For this review, use the dimensioned drawing (mm, ordinates from the lowest corner) and the shaded views. Coordinates: 2 decimals unless noted, no trailing zeros. Write each loop counter-clockwise with the first axis right and the second up, starting at its lowest first coordinate (ties: lowest second). Pieces come first, ordered by that corner, then holes. Notation, with made-up numbers: M 37,-0.5 L 83,-0.5 A29 ccw 83,20.5 Z; hole C 41.25,-34 d8. An arc over 180 degrees is marked long. Return JSON: item names as keys, results as strings. Group by question number.
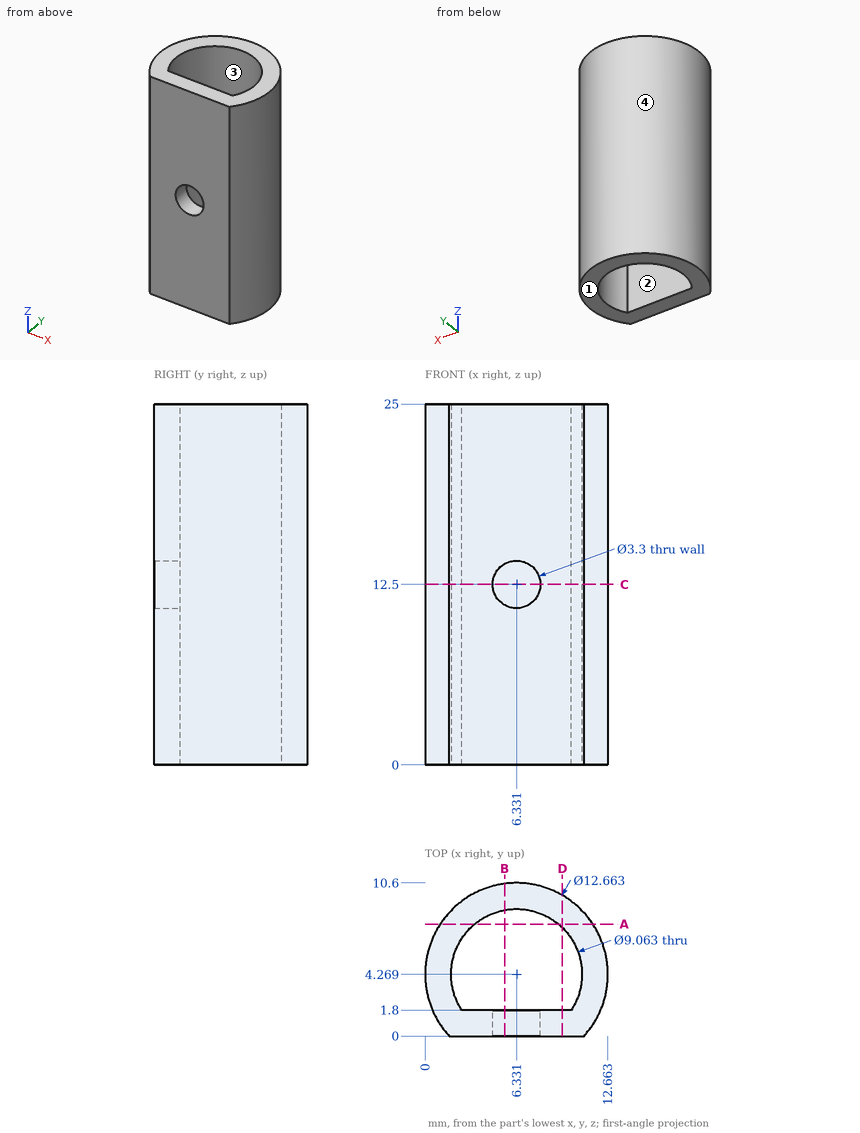
Item 1: The part is to be moulded in two halves that separate along X. For the marked faces 1, 2, 3 and 4, say which applies: pulls with the +X half, pulls with the -X half, needs draft (parallel to the pull), parting line crosses it, or undercut.
Item 2: For pin 1 (1 mm diameter, centred on y = 3, z = 8, fed in from -X), flat-tipped, find the tip position at first contact; note if it passes through.
Item 3: Add section A-A (y = 7.75). Write out the cut boundary in (x, z), plus the area to 3 significant figures.
Item 4: Add section C-C (z = 12.5). Write out the cut boundary in (x, y) (1 decimal).
Item 5: Add section D-D (x = 9.5). Write out the cut boundary in (y, z), plus the area to 3 significant figures.
Item 6: Add section B-B (x = 5.5). Write out the cut boundary in (y, z) (1 decimal).
Item 7: For line 1 (X direction, y = 3.25, z = 17.25) (1 decimal); line 2 (X direction, y = 7.5, z = 21.25) (1 decimal); line 3 (Y direction, x = 9, z = 20.25), list the stretches that pass through material, from the lowest coordinate up.
Geometry check:
{
 "1": {"face 1": "needs draft", "face 2": "undercut", "face 3": "undercut", "face 4": "parting line crosses it"},
 "2": {"pin 1": "x = 0.05"},
 "3": {"outline": "M 1.04,0 L 3.43,0 L 3.43,25 L 1.04,25 Z; M 9.23,0 L 11.62,0 L 11.62,25 L 9.23,25 Z", "area": "119 mm^2"},
 "4": {"outline": "M 1.7,0 L 4.7,0 L 4.7,1.8 L 2.5,1.8 A4.5 cw long 10.1,1.8 L 8,1.8 L 8,0 L 11,0 A6.3 ccw long Z"},
 "5": {"outline": "M 0,0 L 1.8,0 L 1.8,25 L 0,25 Z; M 7.51,0 L 9.75,0 L 9.75,25 L 7.51,25 Z", "area": "101 mm^2"},
 "6": {"outline": "M 0,0 L 1.8,0 L 1.8,11.1 L 0,11.1 Z; M 0,13.9 L 1.8,13.9 L 1.8,25 L 0,25 Z; M 8.7,0 L 10.5,0 L 10.5,25 L 8.7,25 Z"},
 "7": {"line 1": "0.1 to 1.9, 10.7 to 12.6", "line 2": "0.9 to 3.2, 9.5 to 11.8", "line 3": "0 to 1.8, 7.93 to 10.01"}
}
